The figure shows three views and two pictorial views of one solid part (mm, origin at its lowest corner). Answer the questions. Give positions to 0.01 mm unless a question says otherwise; leave off trailing zeros. Write each loop counter-clockwise with the first axis right and the second up, starting at its lowest first coordinate (ties: lowest second). Pieces come first, ordered by that corner, then holes. Notation, with made-up numbers: (39, 54.25) - (51, 54.25) arc R38 ccw to (51, 92.25) - close; hole circle Ø5 at (25, 37.25). An arc over 180 degrees is marked (long way). Answer as CSV lines item,"result". Start each with the question number.
(1) Find section B-B (x = 26.5). Write down the section's boundary in (y, z), then the cut area to 3 significant figures.
(2) Each of these flat-tipped pins is pushed along its axis until it touches: pin 1 Ø5 at (x, z) = (4, 5) entering from +Y; pin 2 Ø3 at (x, y) = (277.5, 11) entering from -Z; pin 3 Ø5 at (y, z) = (10, 9.5) entering from -X. Where does it stop, or does it pass through?
(3) Straight lines are drawn through the part: probe 1 along Z at (x, y) = (195.5, 6.75); probe 2 along X at (y, z) = (10.25, 8.75); probe 3 along Z at (x, y) = (196, 7.25). For each, find the intervals that lie inside material, in ascending order.
(4) Find section A-A (z = 6.35). Write down the section's boundary in (x, y), then the cut area to 3 significant figures.
(5) Find section C-C (y = 10). Write down the section's boundary in (x, z).
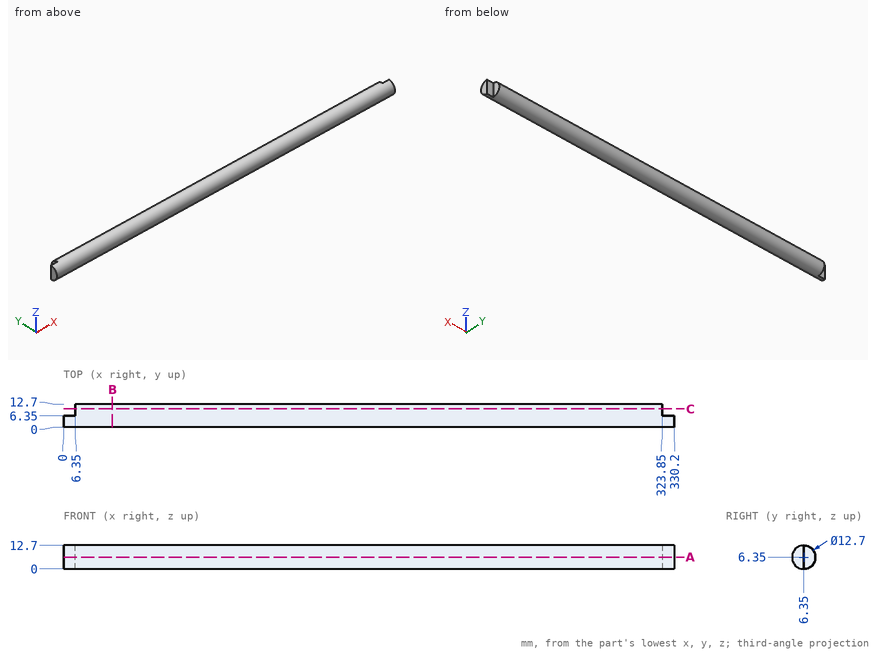
Result set:
1,outline,"circle Ø12.7 at (6.35, 6.35)"
1,area,"127 mm^2"
2,pin 1,"y = 12.68"
2,pin 2,"z = 0.84"
2,pin 3,"x = 6.35"
3,probe 1,"0.01 to 12.69"
3,probe 2,"6.35 to 323.85"
3,probe 3,"0.06 to 12.64"
4,outline,"(0, 0) - (330.2, 0) - (330.2, 6.35) - (323.85, 6.35) - (323.85, 12.7) - (6.35, 12.7) - (6.35, 6.35) - (0, 6.35) - close"
4,area,"4,110 mm^2"
5,outline,"(6.35, 1.15) - (323.85, 1.15) - (323.85, 11.55) - (6.35, 11.55) - close"
